from build123d import *

# Parameters (mm, degrees)
ESQUISSE1_R                   = 11.75
BOSS_EXTRU_1_DEPTH            = 19.4
ESQUISSE2_R                   = 8.2
BOSS_EXTRU_2_DEPTH            = 8.8
ENL_V_START                   = -5.9
ENL_V_MAT_EXTRU_1_OUTLINE_W   = 6.8
ENL_V_MAT_EXTRU_1_OUTLINE_H   = 12.3
ENL_V_MAT_EXTRU_1_DEPTH       = 11.8
ENL_V_START_2                 = -1.8
ENL_V_MAT_EXTRU_1_2_OUTLINE_W = 3.4
ENL_V_MAT_EXTRU_1_2_OUTLINE_H = 12.3
ENL_V_MAT_EXTRU_1_2_DEPTH     = 3.6
ENL_V_START_3                 = -3.2
ENL_V_MAT_EXTRU_1_3_OUTLINE_W = 1.9
ENL_V_MAT_EXTRU_1_3_OUTLINE_H = 12.3
ENL_V_MAT_EXTRU_1_3_DEPTH     = 6.4
BOSS_EXTRU_3_START            = -4.7
BOSS_EXTRU_3_OUTLINE_W        = 28
BOSS_EXTRU_3_OUTLINE_H        = 32.8
BOSS_EXTRU_3_OUTLINE_R        = 1.5
BOSS_EXTRU_3_DEPTH            = 4.7
ESQUISSE5_R                   = 11.25
BOSS_EXTRU_4_DEPTH            = 1.6
BOSS_EXTRU_4_TAPER            = 15
ESQUISSE6_R                   = 9.5
ESQUISSE6_R_2                 = 8
ENL_V_MAT_EXTRU_2_DEPTH       = 13.5
ENL_V_MAT_EXTRU_3_DEPTH       = 12.5
CHANFREIN1_SIZE               = 1.5
CONG_1_R                      = 2.5
ENL_V_MAT_EXTRU_4_DEPTH       = 2.5
ENL_V_MAT_EXTRU_4_DEPTH_BACK  = 35.225502188
ENL_V_MAT_EXTRU_5_DEPTH       = 2.5
ENL_V_MAT_EXTRU_5_DEPTH_BACK  = 35.225502188
ESQUISSE10_W                  = 8
ESQUISSE10_H                  = 5.5
ENL_V_MAT_EXTRU_6_DEPTH       = 5
ESQUISSE11_W                  = 7.8
ESQUISSE11_H                  = 4
BOSS_EXTRU_5_DEPTH            = 7.4
ESQUISSE12_W                  = 7.8
ESQUISSE12_H                  = 6
BOSS_EXTRU_6_DEPTH            = 2.5
CHANFREIN2_SIZE               = 0.5


# Read off the part's stored shape, not the designer's step: Enlèv. mat.-Extru.1, Boss.-Extru.3
with BuildPart() as part:
    # Esquisse1 → Boss.-Extru.1 (new body)
    with BuildSketch(Plane.XY):
        Circle(ESQUISSE1_R)
    extrude(amount=BOSS_EXTRU_1_DEPTH)

    # Esquisse2 → Boss.-Extru.2 (add)
    with BuildSketch(Plane.XY.offset(19.4)):
        Circle(ESQUISSE2_R)
    extrude(amount=BOSS_EXTRU_2_DEPTH)

    # Enlèv. mat.-Extru.1 outline → Enlèv. mat.-Extru.1 (cut)
    with BuildSketch(Plane.YZ.offset(ENL_V_START)):
        with Locations((-0.2, 22.05)):
            Rectangle(ENL_V_MAT_EXTRU_1_OUTLINE_W, ENL_V_MAT_EXTRU_1_OUTLINE_H)
    extrude(amount=ENL_V_MAT_EXTRU_1_DEPTH, mode=Mode.SUBTRACT)

    # Enl_v. mat.-Extru.1 2 outline → Enl_v. mat.-Extru.1 2 (cut)
    with BuildSketch(Plane.YZ.offset(ENL_V_START_2)):
        with Locations((-5.3, 22.05)):
            Rectangle(ENL_V_MAT_EXTRU_1_2_OUTLINE_W, ENL_V_MAT_EXTRU_1_2_OUTLINE_H)
    extrude(amount=ENL_V_MAT_EXTRU_1_2_DEPTH, mode=Mode.SUBTRACT)

    # Enl_v. mat.-Extru.1 3 outline → Enl_v. mat.-Extru.1 3 (cut)
    with BuildSketch(Plane.YZ.offset(ENL_V_START_3)):
        with Locations((-4.55, 22.05)):
            Rectangle(ENL_V_MAT_EXTRU_1_3_OUTLINE_W, ENL_V_MAT_EXTRU_1_3_OUTLINE_H)
    extrude(amount=ENL_V_MAT_EXTRU_1_3_DEPTH, mode=Mode.SUBTRACT)

    # Boss.-Extru.3 outline → Boss.-Extru.3 (add)
    with BuildSketch(Plane.XY.offset(BOSS_EXTRU_3_START)):
        Rectangle(BOSS_EXTRU_3_OUTLINE_W, BOSS_EXTRU_3_OUTLINE_H)
        with Locations((-9.5, -11.9)):
            Circle(BOSS_EXTRU_3_OUTLINE_R, mode=Mode.SUBTRACT)
        with Locations((9.5, 11.9)):
            Circle(BOSS_EXTRU_3_OUTLINE_R, mode=Mode.SUBTRACT)
    extrude(amount=BOSS_EXTRU_3_DEPTH)

    # Esquisse5 → Boss.-Extru.4 (add)
    with BuildSketch(Plane(origin=(0, 0, -4.7), x_dir=(-1, 0, 0), z_dir=(0, 0, -1))):
        Circle(ESQUISSE5_R)
    extrude(amount=BOSS_EXTRU_4_DEPTH, taper=BOSS_EXTRU_4_TAPER)

    # Esquisse6 → Enlèv. mat.-Extru.2 (cut)
    with BuildSketch(Plane(origin=(0, 0, -6.3), x_dir=(-1, 0, 0), z_dir=(0, 0, -1))):
        Circle(ESQUISSE6_R)
        Circle(ESQUISSE6_R_2, mode=Mode.SUBTRACT)
    extrude(amount=-ENL_V_MAT_EXTRU_2_DEPTH, mode=Mode.SUBTRACT)

    # Esquisse7 → Enlèv. mat.-Extru.3 (cut)
    with BuildSketch(Plane(origin=(0, 0, -6.3), x_dir=(-1, 0, 0), z_dir=(0, 0, -1))):
        Polygon((-3.2, 3.4), (-3.2, 5.3), (-1.8, 5.3), (-1.8, 6.8), (1.8, 6.8), (1.8, 5.3), (3.2, 5.3), (3.2, 3.4), (5.9, 3.4), (5.9, -3.4), (-5.9, -3.4), (-5.9, 3.4), align=None)
    extrude(amount=-ENL_V_MAT_EXTRU_3_DEPTH, mode=Mode.SUBTRACT)

    # Chanfrein1
    chanfrein1_edges = [part.edges().sort_by_distance(p)[0] for p in [
        (8, 11.9, -4.7),
        (-11, -11.9, -4.7),
    ]]
    chamfer(chanfrein1_edges, length=CHANFREIN1_SIZE)

    # Congé1
    cong_1_edges = [part.edges().sort_by_distance(p)[0] for p in [
        (14, 16.4, -2.35),
        (14, -16.4, -2.35),
        (-14, -16.4, -2.35),
        (-14, 16.4, -2.35),
    ]]
    fillet(cong_1_edges, radius=CONG_1_R)

    # Esquisse8 → Enlèv. mat.-Extru.4 (cut, two sides: drawn at the far end of the back side and taken through both)
    with BuildSketch(Plane(origin=(-4.65, 0, 4.65), x_dir=(0, 1, 0), z_dir=(0.7071067811865464, 0, -0.7071067811865488)).offset(-ENL_V_MAT_EXTRU_4_DEPTH_BACK)):
        with BuildLine():
            Line((-11.4, -13.222896808), (11.4, -13.222896808))
            ThreePointArc((11.4, -13.222896808), (0, -11.922896808), (-11.4, -13.222896808))
        make_face()
    extrude(amount=ENL_V_MAT_EXTRU_4_DEPTH + ENL_V_MAT_EXTRU_4_DEPTH_BACK, mode=Mode.SUBTRACT)

    # Esquisse9 → Enlèv. mat.-Extru.5 (cut, two sides: drawn at the far end of the back side and taken through both)
    with BuildSketch(Plane(origin=(4.65, 0, 4.65), x_dir=(0, -1, 0), z_dir=(-0.7071067811865464, 0, -0.7071067811865488)).offset(-ENL_V_MAT_EXTRU_5_DEPTH_BACK)):
        with BuildLine():
            Line((-11.4, -13.222896808), (11.4, -13.222896808))
            ThreePointArc((11.4, -13.222896808), (0, -11.922896808), (-11.4, -13.222896808))
        make_face()
    extrude(amount=ENL_V_MAT_EXTRU_5_DEPTH + ENL_V_MAT_EXTRU_5_DEPTH_BACK, mode=Mode.SUBTRACT)

    # Esquisse10 → Enlèv. mat.-Extru.6 (cut)
    with BuildSketch(Plane(origin=(0, 0, -6.3), x_dir=(-1, 0, 0), z_dir=(0, 0, -1))):
        with Locations((0, -11.25)):
            Rectangle(ESQUISSE10_W, ESQUISSE10_H)
    extrude(amount=-ENL_V_MAT_EXTRU_6_DEPTH, mode=Mode.SUBTRACT)

    # Esquisse11 → Boss.-Extru.5 (add)
    with BuildSketch(Plane(origin=(0, 0, -1.3), x_dir=(-1, 0, 0), z_dir=(0, 0, -1))):
        with Locations((0, -11.9)):
            Rectangle(ESQUISSE11_W, ESQUISSE11_H)
    extrude(amount=BOSS_EXTRU_5_DEPTH)

    # Esquisse12 → Boss.-Extru.6 (add)
    with BuildSketch(Plane(origin=(0, 0, -8.7), x_dir=(-1, 0, 0), z_dir=(0, 0, -1))):
        with Locations((0, -12.9)):
            Rectangle(ESQUISSE12_W, ESQUISSE12_H)
    extrude(amount=BOSS_EXTRU_6_DEPTH)

    # Chanfrein2
    chanfrein2_edges = [part.edges().sort_by_distance(p)[0] for p in [
        (5.9, -0.2, 28.2),
        (0, 3.2, 28.2),
        (-5.9, -0.2, 28.2),
        (5.9, 0, -6.3),
        (0, -3.4, -6.3),
        (-5.9, 0, -6.3),
    ]]
    chamfer(chanfrein2_edges, length=CHANFREIN2_SIZE)


solid = part.part
Input: part model. Units: mm. Frame: model coordinates. A direction names the side the tool comes from. Coordinates: 2 decimals unless noted, no trailing zeros. Loops run counter-clockwise (first coordinate to the right, second up) from the corner with the lowest first, then second, coordinate; pieces in that order, holes last. Notation, with made-up numbers: (11, -23.75) -> (24, -23.75) arc R30 ccw to (24, 13.25) -> close; hole circle Ø9 at (74, 84.25). An arc over 180 degrees is marked (long way). Write item = value, one per line. Start each with the question number.
Item 1: First-contact query: P1, Ø5, axis at x = 9.5, y = 11.9, coming from the -Z side; P2, Ø3, axis at x = 0, z = -10, coming from the -Y side; P3, Ø15, axis at x = -3.5, y = 3.5, coming from the -Z side. Flat tips, straight axial feed; report the tip coordinate or a pass-through.
Item 2: Reachability of faces 4 (the face through (0, -15, -8.7)), 5 (the face through (0, -15.9, -10)), 6 (the face through (5.9, 0, 0)), 7 (the face through (0, -13.9, -5)), 8 (the face through (5, -3.6, 22)) from +Z, -Z, +X, -X, +Y, -Y: full face, straight path, thin tool, end or side. Return the list, or none.
Item 3: Cut plane B-B, the plane z = 11.5. Return loops of the section in (x, y), plus the area to 3 significant figures.
Item 4: Material intervals for line 1 (Y direction, x = 0, z = 4); line 2 (Y direction, x = 4.75, z = 2); line 3 (Y direction, x = 1.5, z = 6.5), sorted ascending.
Item 5: Mould query, pull axis X, two halves, no side actions, for faces 1 (the face through (0, -7, 22)), 2 (the face through (0, -5, -6.3)), 3 (the face through (-13.287, 15.648, -2.317)). Classes: pulls with the +X half, pulls with the -X half, needs draft (parallel to the pull), parting line crosses it, or undercut.
Item 6: Cut plane A-A, the plane z = 4.5. Return loops of the section in (x, y).
Ans:
q1.P1 = -4.2
q1.P2 = -15.9
q1.P3 = -6.3
q2.face_4 = +X, -X, -Y
q2.face_5 = -Z, +X, -X, -Y
q2.face_6 = -Z
q2.face_7 = none
q2.face_8 = +Z
q3.outline = circle Ø23.5 at (0, 0)
q3.area = 434 mm²
q4.line_1 = -11.75 to -9.5, -8 to -3.4, 6.8 to 8, 9.5 to 11.75
q4.line_2 = -10.75 to -8.23, -6.44 to -3.4, 3.4 to 6.44, 8.23 to 10.75
q4.line_3 = -11.65 to -9.38, -7.86 to 7.86, 9.38 to 11.65
q5.face_1 = undercut
q5.face_2 = needs draft
q5.face_3 = pulls with the -X half
q6.outline = circle Ø23.5 at (0, 0); circle Ø16 at (0, 0); hole circle Ø19 at (0, 0); hole (-5.9, -3.4) -> (5.9, -3.4) -> (5.9, 3.4) -> (3.2, 3.4) -> (3.2, 5.3) -> (1.8, 5.3) -> (1.8, 6.8) -> (-1.8, 6.8) -> (-1.8, 5.3) -> (-3.2, 5.3) -> (-3.2, 3.4) -> (-5.9, 3.4) -> close
